Input: part model. Units: mm. Frame: model coordinates. Face numbers are marked on the shaded views. A direction names the side the tool comes from. Give positions to 0.01 mm unless a question says otherwise; leave off trailing zeros. Write each loop counter-clockwise with the first axis right and the second up, starting at its lowest first coordinate (ties: lowest second). Pieces come first, ordered by that corner, then holes.
```python
from build123d import *

# Parameters (mm, degrees)
PAD005_DEPTH            = 1
PAD006_DEPTH            = 11
SKETCH007_R             = 0.45
POCKET_DEPTH            = 10
BODY003_PLACEMENT_ANGLE = 90


with BuildPart() as part:
    # Sketch005 → Pad005 (new body)
    with BuildSketch(Plane.XY):
        Polygon((0, -11), (3.5, -7.5), (3.5, 7.5), (0, 11), (-3.5, 7.5), (-3.5, -7.5), align=None)
    extrude(amount=PAD005_DEPTH)

    # Sketch006 (on Face8 of Pad005) → Pad006 (join)
    with BuildSketch(Plane.XY.offset(1)):
        Polygon((-2, -3), (1.973969, -3), (2, -7), (-2, -7), align=None)
    extrude(amount=PAD006_DEPTH)

    # Sketch007 (on Face12 of Pad006) → Pocket (cut)
    with BuildSketch(Plane(origin=(0, -3, 0), x_dir=(-1, 0, 0), z_dir=(0, 1, 0))):
        with Locations((0, 9)):
            Circle(SKETCH007_R)
    extrude(amount=-POCKET_DEPTH, mode=Mode.SUBTRACT)


with BuildPart() as part_1:
    # Body003 placement: moved
    add(part.part.moved(Location((0, 9, -2))).rotate(Axis((0, 9, -2), (1, 0, 0)), BODY003_PLACEMENT_ANGLE))


solid = part_1.part
```
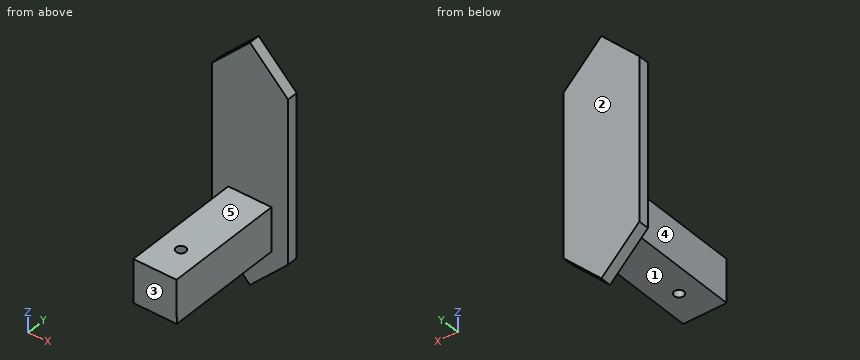
Q1. Access query for the marked faces 4 and 5. Directions: +Z, -Z, +X, -X, +Y, -Y. A direction counts if a zero-diameter tool reaches every point of the face in a straight line with its end or side. Return the directions, or none.
Q2. Mould query, pull axis Y, two halves, no side actions, for the marked faces 1, 2 and 3. Classes: +Y half, -Y half, draft (parallel to the pull), parting line (faces both ways), or undercut.
Q3. Section A-A, the plane y = 0. Return the cut outline in (x, z).
Q4. Section C-C, the plane z = -7.5. Return the cut outline in (x, y).
Q5. Section B-B, the plane x = 1.25. Return the cut outline in (y, z).
Q6. Pin query (flat end, axial travel): pin 1 (2 mm diameter, centred on x = -2.5, y = 1.5, fed in from -Z); pin 2 (1.2 mm diameter, centred on x = 0, y = 0.5, fed in from +Z); pin 3 (2 mm diameter, centred on y = 4.5, z = -7.5, fed in from -X). Return the tip coordinate at first contact, or that it passes through.
Q7. Material intervals for line 1 along Y through (x, z) = (0, -7.45); line 2 along Z through (x, y) = (0.25, 6.5); line 3 along X through (y, z) = (0, -6.55), sorted ascending.
Q8. Section D-D, the plane z = 4.5. Return the cut outline in (x, y), then the cut area to 3 significant figures.
Solutions:
1. face 4: +Z, -Z, -X, -Y
1. face 5: +Z, +X, -X, -Y
2. face 1: draft
2. face 2: +Y half
2. face 3: -Y half
3. outline: (-2, -9) - (-0.45, -9) - (-0.45, -5) - (-2, -5) - close; (0.45, -9) - (2, -9) - (1.97, -5) - (0.45, -5) - close
4. outline: (-3.5, 8) - (-2, 8) - (-2, -3) - (1.99, -3) - (1.99, 8) - (3.5, 8) - (3.5, 9) - (-3.5, 9) - close; hole circle Ø0.9 at (0, 0)
5. outline: (-3, -9) - (8, -9) - (8, -11.75) - (9, -11.75) - (9, 7.75) - (8, 7.75) - (8, -5) - (-3, -5) - close
6. pin 1: stops at z = -9
6. pin 2: stops at z = -5
6. pin 3: stops at x = -2
7. line 1: y = -3 to -0.45, 0.45 to 9
7. line 2: z = -9 to -5
7. line 3: x = -2 to -0.45, 0.45 to 1.98
8. outline: (-3.5, 8) - (3.5, 8) - (3.5, 9) - (-3.5, 9) - close
8. area: 7.00 mm2
